Design review of the part shown in the three views and the two pictorial views. Dimensions are in mm from the part's minimum x, y and z. Round coordinates to 2 decimals unless told otherwise and drop trailing zeros. Loops run counter-clockwise (first coordinate to the right, second up) from the corner with the lowest first, then second, coordinate; pieces in that order, holes last. Notation, with made-up numbers: M 81,-27 L 138,-27 A6 cw 138,-22 Z; hole C 40,26 d10. An arc over 180 degrees is marked long. One line per question, with ' | ' between items. Start each with the question number.
1) For pin 1 Ø4.5 at (x, z) = (44.45, 10.4) entering from +Y, flat-tipped, find the tip position at first contact; note if it passes through.
2) We need section B-B (x = 44.45). Give the boundary of the cut face in (y, z) (1 decimal).
3) We need section A-A (z = 25.4). Give the boundary of the cut face in (x, y), and give its area (3 significant figures).
4) We need section C-C (y = 5.5). State how many separate pieces and enclosed holes the cut face has, and give its area (3 significant figures).
5) For probe 1 along Z at (x, y) = (44.45, 13.5) (1 decimal); probe 2 along Z at (x, y) = (12.5, 16.25); probe 3 along Z at (x, y) = (9.5, 12), list the stretches that pass through material, from the lowest coordinate up. Write a range as from..to.
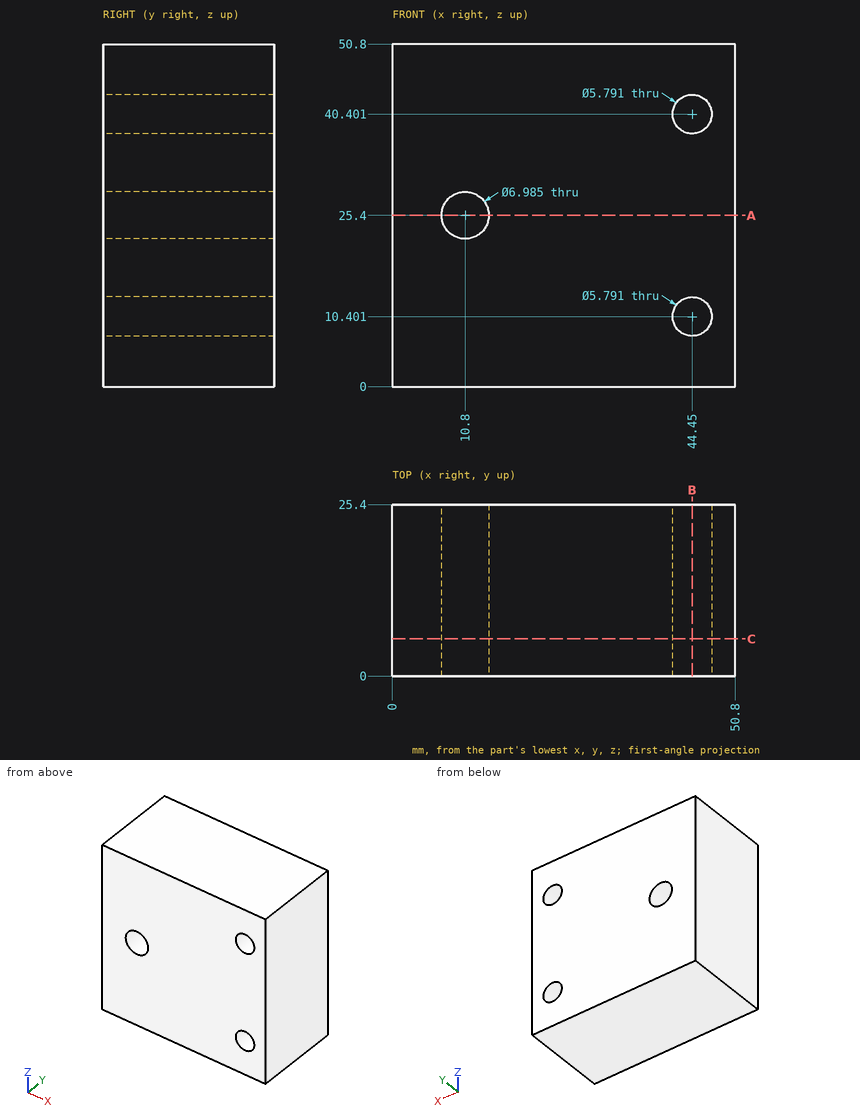
Answers below:
1) pin 1: through
2) outline: M 0,0 L 25.4,0 L 25.4,7.5 L 0,7.5 Z; M 0,13.3 L 25.4,13.3 L 25.4,37.5 L 0,37.5 Z; M 0,43.3 L 25.4,43.3 L 25.4,50.8 L 0,50.8 Z
3) outline: M 0,0 L 7.31,0 L 7.31,25.4 L 0,25.4 Z; M 14.29,0 L 50.8,0 L 50.8,25.4 L 14.29,25.4 Z | area: 1,110 mm^2
4) separate pieces: 1 | enclosed holes: 3 | area: 2,490 mm^2
5) probe 1: 0..7.5, 13.3..37.5, 43.3..50.8 | probe 2: 0..22.35, 28.45..50.8 | probe 3: 0..22.16, 28.64..50.8
